from build123d import *

# Parameters (mm, degrees)
SKETCH_1_W          = 6
SKETCH_1_H          = 24
SKETCH_1_W_2        = 45
SKETCH_1_H_2        = 6
EXTRUDE_1_DEPTH     = 30
FILLET_1_R          = 15
CUT_EXTRUDE_1_REACH = 74.312
SKETCH_2_R          = 6
CUT_EXTRUDE_2_DEPTH = 54.686590505


with BuildPart() as part:
    # Эскиз1 → Бобышка-Вытянуть1 (new body)
    with BuildSketch(Plane.XY):
        with Locations((-34.5, 9)):
            Rectangle(SKETCH_1_W, SKETCH_1_H)
        Polygon((-31.5, 21), (-22.5, 21), (-22.5, 27), (-37.5, 27), (-37.5, 21), align=None)
        Polygon((-22.5, 21), (-22.5, 3), (-16.5, 3), (-16.5, 27), (-22.5, 27), align=None)
        Rectangle(SKETCH_1_W_2, SKETCH_1_H_2)
    extrude(amount=EXTRUDE_1_DEPTH)

    # Скругление1
    fillet_1_edges = [part.edges().sort_by_distance(p)[0] for p in [
        (-34.5, -3, 0),
        (-34.5, -3, 30),
    ]]
    fillet(fillet_1_edges, radius=FILLET_1_R - 0.0001)  # a hair under: the kernel refuses the full size

    # Эскиз2 → Вырез-Вытянуть1 (cut, up to next)
    with BuildSketch(Plane.ZY.offset(37.5), mode=Mode.PRIVATE) as cut_extrude_1_sk1:
        with Locations((15, 12)):
            Circle(SKETCH_2_R)
    cut_extrude_1_tool1 = extrude(cut_extrude_1_sk1.sketch, amount=-CUT_EXTRUDE_1_REACH, mode=Mode.PRIVATE) & part.part
    add(cut_extrude_1_tool1.solids().sort_by_distance((-37.5, 12, 15))[0], mode=Mode.SUBTRACT)

    # Эскиз3 → Вырез-Вытянуть2 (cut, through all)
    with BuildSketch(Plane(origin=(0, 3, 0), x_dir=(1, 0, 0), z_dir=(0, 1, 0))):
        with BuildLine():
            Line((22.5, -7.5), (11.5, -7.5))
            ThreePointArc((11.5, -7.5), (4, -15), (11.5, -22.5))
            Line((11.5, -22.5), (22.5, -22.5))
            Line((22.5, -22.5), (22.5, -7.5))
        make_face()
    extrude(amount=-CUT_EXTRUDE_2_DEPTH, mode=Mode.SUBTRACT)


solid = part.part
Design review of the part built by this model. Coordinates are the model's own, in mm. A direction names the side the tool comes from. Round coordinates to 2 decimals unless told otherwise and drop trailing zeros. Write each loop counter-clockwise with the first axis right and the second up, starting at its lowest first coordinate (ties: lowest second). Pieces come first, ordered by that corner, then holes. Notation, with made-up numbers: (-1, 85) - (24, 85) arc R20 cw to (24, 99) - close; hole circle Ø4 at (-6, -14.5). An arc over 180 degrees is marked (long way). Use a Markdown table: item, result. Add a question column.
1. We need section C-C (y = 14). State the section outline as (x, z) points.
2. Wall thickness on probe 1 along X at (y, z) = (5, 10); probe 2 along Y at (x, z) = (-36.2, 15); probe 3 along X at (y, z) = (7.5, 13.5): over which ranges is each line inside the solid? List them lowest first.
3. Mouldability with a two-part tool opening along Y and no side actions: class faces 1 (the face through (-2, 3, 15)), 2 (the face through (-16.5, 15, 15)), 3 (the face through (-34.54, 9.7, 20.54)) as +Y half, -Y half, draft (parallel to the pull), parting line (faces both ways), or undercut.
4. Clearance check with flat-ended pins moving along their axes: pin 1 (12 mm diameter, centred on y = 18, z = 8, fed in from +X); pin 2 (3 mm diameter, centred on x = 8.5, z = 9, fed in from -Y); pin 3 (9.5 mm diameter, centred on y = 12, z = 15, fed in from -X); pin 4 (9 mm diameter, centred on x = 7, z = 10.5, fed in from +Y). State where each tip first meets the part, or that it passes through.
5. We need section B-B (z = 16). State the section outline as (x, y) points.
6. For faces 4 (the face through (-22.5, 9, 15)), 5 (the face through (-34.46, 1.28, 4.51)), 6 (the face through (-34.46, 1.28, 25.49)), 7 (the face through (17, 0, 22.5)), list the 3-axis set-ups (+Z, -Z, +X, -X, +Y, -Y) from which the entire face can be reached by the end or side of a thin tool; tool diameter is ignored.
7. We need section A-A (x = 19.5). State the section outline as (y, z) points.
8. We need section D-D (y = 5). State the section outline as (x, z) points.
Output:
| question | item | result |
|---|---|---|
| 1 | outline | (-37.5, 0) - (-31.5, 0) - (-31.5, 9.34) - (-37.5, 9.34) - close; (-37.5, 20.66) - (-31.5, 20.66) - (-31.5, 30) - (-37.5, 30) - close; (-22.5, 0) - (-16.5, 0) - (-16.5, 30) - (-22.5, 30) - close |
| 2 | probe 1 | x = -37.5 to -31.5, -22.5 to -16.5 |
| 2 | probe 2 | y = -3 to 6, 18 to 27 |
| 2 | probe 3 | x = -22.5 to -16.5 |
| 3 | face 1 | +Y half |
| 3 | face 2 | draft |
| 3 | face 3 | undercut |
| 4 | pin 1 | stops at x = -16.5 |
| 4 | pin 2 | stops at y = -3 |
| 4 | pin 3 | stops at x = -22.5 |
| 4 | pin 4 | stops at y = 3 |
| 5 | outline | (-37.5, -2.97) - (-31.5, -2.97) - (-31.5, 6.08) - (-37.5, 6.08) - close; (-37.5, 17.92) - (-31.5, 17.92) - (-31.5, 21) - (-22.5, 21) - (-22.5, -3) - (4.07, -3) - (4.07, 3) - (-16.5, 3) - (-16.5, 27) - (-37.5, 27) - close |
| 6 | face 4 | +Z, -Z, -Y |
| 6 | face 5 | -Z, -X, -Y |
| 6 | face 6 | +Z, -X, -Y |
| 6 | face 7 | +X, +Y, -Y |
| 7 | outline | (-3, 0) - (3, 0) - (3, 7.5) - (-3, 7.5) - close; (-3, 22.5) - (3, 22.5) - (3, 30) - (-3, 30) - close |
| 8 | outline | (-37.5, 1.73) - (-31.5, 1.73) - (-31.5, 28.27) - (-37.5, 28.27) - close; (-22.5, 0) - (-16.5, 0) - (-16.5, 30) - (-22.5, 30) - close |
